from build123d import *

# Parameters (mm, degrees)
F0_W      = 20
F0_H      = 8
F1_DEPTH  = 1
F3_DEPTH  = 5.5
F4_R      = 2.5
F5_R      = 3.0047096082
F6_R      = 1.2
F7_W      = 20
F7_H      = 1.5
F8_DEPTH  = 25
F9_R      = 1.6945445142
F10_DEPTH = 25


with BuildPart() as f1:
    # F0 (on Front) → F1 (new body)
    with BuildSketch(Plane.XZ):
        with Locations((-0.9586364031, -3.9746239682)):
            Rectangle(F0_W, F0_H)
    extrude(amount=F1_DEPTH)

    # F2 (on face) → F3 (join)
    with BuildSketch(Plane.XZ.offset(1)):
        Polygon((7.0413635969, 0.0253760318), (-8.9586364031, 0.0253760318), (-7.2086364031, -6.4746239682), (5.2913635969, -6.4746239682), align=None)
    extrude(amount=F3_DEPTH)

    # F4
    f4_edges = [f1.edges().sort_by_distance(p)[0] for p in [
        (7.041364, -3.75, 0.025376),
        (-8.958636, -3.75, 0.025376),
    ]]
    fillet(f4_edges, radius=F4_R)

    # F5
    f5_edges = [f1.edges().sort_by_distance(p)[0] for p in [
        (5.291364, -3.75, -6.474624),
        (-7.208636, -3.75, -6.474624),
    ]]
    fillet(f5_edges, radius=F5_R)

    # F6
    f6_edges = [f1.edges().sort_by_distance(p)[0] for p in [
        (6.04166, -6.5, -3.687808),
        (4.816347, -6.5, -5.854804),
        (5.763558, -6.5, -0.953906),
        (-0.958636, -6.5, -6.474624),
        (-0.958636, -6.5, 0.025376),
        (-6.73362, -6.5, -5.854804),
        (-7.680831, -6.5, -0.953906),
        (-7.958933, -6.5, -3.687808),
    ]]
    fillet(f6_edges, radius=F6_R)

    # F7 (on face) → F8 (cut)
    with BuildSketch(Plane.XZ.offset(1)):
        with Locations((-0.9586364031, -7.2246239682)):
            Rectangle(F7_W, F7_H)
    extrude(amount=-F8_DEPTH, mode=Mode.SUBTRACT)

    # F9 (on face) → F10 (cut)
    with BuildSketch(Plane.XZ.offset(1)):
        with Locations((9.0413635969, 0.0253760318)):
            Circle(F9_R)
    extrude(amount=-F10_DEPTH, mode=Mode.SUBTRACT)


solid = f1.part
The model under review builds one solid part; all positions refer to its coordinate system, in mm. A direction names the side the tool comes from. Coordinates: 2 decimals unless noted, no trailing zeros. Loops run counter-clockwise (first coordinate to the right, second up) from the corner with the lowest first, then second, coordinate; pieces in that order, holes last.
(1) Consider section B-B, the plane x = -9. Give the boundary of the cut face in (y, z), plus the area to 3 significant figures.
Determined:
outline: (-1, -6.47) - (0, -6.47) - (0, 0.03) - (-1, 0.03) - close
area: 6.50 mm2
(2) Consider section C-C, the plane y = -4.75. Give the boundary of the cut face in (x, z), plus the area to 3 significant figures.
Determined:
outline: (-8.11, -3.12) - (-7.81, -4.25) arc R3 ccw to (-4.91, -6.47) - (2.99, -6.47) arc R3 ccw to (5.89, -4.25) - (6.19, -3.12) arc R2.5 ccw to (3.78, 0.03) - (-5.7, 0.03) arc R2.5 ccw to start
area: 85.7 mm2
(3) Tool access review of faces 1 (the cylindrical face through (-6.8, -3.2, -5.8)), 2 (the cylindrical face through (4.794, -3.18, -5.871)), 3 (the flat face through (-2, -2, 0.025)): name each direction out of +Z, -Z, +X, -X, +Y, -Y from which nothing blocks a thin tool from reaching the whole face with its end or side.
Determined:
face 1: -Z, -X, -Y
face 2: -Z, +X, -Y
face 3: +Z, +X, -X, +Y, -Y
(4) Wall thickness on L1, parallel to Y at x = -7.25, z = -6; L2, parallel to Y at x = 0.25, z = -5.5; L3, parallel to X at y = -1.25, z = -2.5: over which ranges is each line inside the solid? List them lowest first.
Determined:
L1: y = -1 to 0
L2: y = -6.48 to 0
L3: x = -8.2 to 6.28
(5) Insertion check: P1, Ø3, axis at x = 7, z = -2.5, coming from the -Y side. The pin has a flat end and moves straight along its axis. Give the tip position at first contact, or say it passes through.
Determined:
P1: stops at y = -6.42
(6) Consider section A-A, the plane y = -0.75. Give the boundary of the cut face in (x, z).
Determined:
outline: (-10.96, -6.47) - (9.04, -6.47) - (9.04, -1.67) arc R1.69 cw to (7.35, 0.03) - (-10.96, 0.03) - close
